Autodesk Inventor part; units mm, degrees
ref_plane "YZ Plane" through (0, 0, 0) normal (1, 0, 0) x (0, 1, 0)
ref_plane "XZ Plane" through (0, 0, 0) normal (0, 1, 0) x (-1, 0, 0)
ref_plane "XY Plane" through (0, 0, 0) normal (0, 0, 1) x (1, 0, 0)
sketch "スケッチ1" plane through (0, 0, 0) normal (0, 1, 0) x (-1, 0, 0)
  line L0 (0, 0) -> (54, 0)
  line L1 (54, 0) -> (54, -66.8)
  line L2 (54, -66.8) -> (0, -66.8)
  line L3 (0, -66.8) -> (0, 0)
  dimension "d0" = 54
  dimension "d1" = 66.8
extrude "押し出し1" add sketch "スケッチ1" along normal blind 10
sketch "スケッチ2" plane through (0, 10, 0) normal (0, 1, 0) x (1, 0, 0)
  line L0 (-54, 66.8) -> (-54, 0)
  line L1 (-54, 0) -> (0, 0)
  line L2 (-27, 0) -> (-27, 66.8)
  line L3 (0, 66.8) -> (-54, 66.8)
  line L4 (-54, 33.4) -> (0, 33.4)
  line L5 (0, 0) -> (0, 66.8)
  line L6 (-27, 33.4) -> (-37.15, 33.4)
  line L7 (-37.15, 33.4) -> (-37.15, 53.55)
  line L8 (-37.15, 53.55) -> (-27, 53.55)
  line L9 (-27, 53.55) -> (-27, 33.4)
  line L10 (-37.15, 33.4) -> (-37.15, 13.25)
  line L11 (-37.15, 13.25) -> (-27, 13.25)
  line L12 (-16.85, 33.4) -> (-16.85, 53.55)
  line L13 (-16.85, 53.55) -> (-27, 53.55)
  line L14 (-16.85, 33.4) -> (-16.85, 13.25)
  line L15 (-16.85, 13.25) -> (-27, 13.25)
  dimension "d7" = 20.15
  dimension "d8" = 10.15
extrude "押し出し2" add sketch "スケッチ2" along normal blind 40 contours L3 L2 L8 L7 L4 L0 | L4 L10 L11 L2 L1 L0 | L3 L5 L4 L12 L13 L2 | L2 L15 L14 L4 L5 L1
fillet "フィレット1" radius 5 4 edges at (0, 25, 0) (0, 25, -66.8) (-54, 25, -66.8) (-54, 25, 0)
sketch "スケッチ3" plane through (0, 0, -5) normal (1, 0, 0) x (0, 0, -1)
  line L0 (48.55, 50) -> (8.25, 50)
  line L1 (28.4, 50) -> (28.4, 0)
  line L2 (0, 0) -> (56.8, 0)
  line L3 (18.4, 50) -> (18.4, 0)
  line L4 (0, 50) -> (0, 0)
  line L5 (0, 10) -> (62, 10)
  line L6 (8.25, 10) -> (48.55, 10)
  point P0 (-5, 0)
  point P1 (18.4, 20)
  point P2 (18.4, 40)
  point P3 (38.4, 20)
  point P4 (38.4, 40)
  dimension "d12" = 10
  dimension "d13" = 10
  dimension "d14" = 10
  dimension "d15" = 20
hole "穴1" at (0, 20, -23.4) at (0, 40, -23.4) at (0, 40, -43.4) at (0, 20, -43.4) direction (-1, 0, 0) diameter 3.3 end through all
sketch "スケッチ4" plane through (0, 0, 0) normal (0, -1, 0) x (1, 0, 0)
  line L0 (-5, -66.8) -> (-49, -66.8)
  line L1 (-27, -66.8) -> (-27, 0)
  line L2 (-49, 0) -> (-5, 0)
  line L3 (-54, -61.8) -> (-54, -5)
  line L4 (-54, -33.4) -> (0, -33.4)
  line L5 (0, -5) -> (0, -61.8)
  point P0 (0, 0)
  point P1 (-27, -43.4)
  point P2 (-27, -23.4)
  dimension "d23" = 10
  dimension "d24" = 10
hole "穴2" at (-27, 0, -43.4) at (-27, 0, -23.4) direction (0, 1, 0) diameter 4.1 end through all
fillet "フィレット2" radius 1 4 edges at (-37.15, 50, -33.4) (-27, 50, -13.25) (-16.85, 50, -33.4) (-27, 50, -53.55)
sketch "スケッチ5" plane through (0, 0, 0) normal (0, -1, 0) x (1, 0, 0)
  circle A0 centre (-27, -23.4) radius 2.05
  circle A1 centre (-27, -43.4) radius 2.05
  line L0 (-27, -23.4) -> (-27, -43.4)
  line L1 (-27, -33.4) -> (-18, -33.4)
  line L2 (-18, -33.4) -> (-18, -40.4)
  line L3 (-18, -40.4) -> (-27, -40.4)
  line L4 (-27, -40.4) -> (-27, -33.4)
  line L5 (-18, -33.4) -> (-18, -26.4)
  line L6 (-18, -26.4) -> (-27, -26.4)
  line L7 (-36, -33.4) -> (-36, -40.4)
  line L8 (-36, -40.4) -> (-27, -40.4)
  line L9 (-36, -33.4) -> (-36, -26.4)
  line L10 (-36, -26.4) -> (-27, -26.4)
  point P0 (0, 0)
  dimension "d33" = 7
  dimension "d34" = 9
extrude "押し出し3" cut sketch "スケッチ5" against normal blind 10 contours L6 L5 L1 L0 | L0 L8 L7 L9 L10 | L1 L2 L3 L0
properties part number "framefixpart1_v2"
Work out the finished part from the listing and answer in its coordinate system (mm). A direction names the side the tool comes from. Coordinates: 2 decimals unless noted, no trailing zeros. Order: outer loops, then holes, each group sorted by start corner. A loop starts at its lowest first (then second) coordinate and runs counter-clockwise, first axis right, second up. Notation, with made-up numbers: (25, -29.5) - (52, -29.5) arc R13 ccw to (52, -6.5) - close; hole circle Ø7 at (78, 74.5). An arc over 180 degrees is marked (long way). Answer as a JSON object with one key per item and string values.
1. The mould has two halves that part along Z. Classify faces 4 (the face through (-45.69, 38.61, -24.29)), 5 (the face through (-27, 25, 0)), 6 (the face through (-17.8, 10, -33.1)), 7 (the face through (-1.43, 25.35, -65.3)): +Z half, -Z half, draft (parallel to the pull), parting line (faces both ways), or undercut.
Output values:
{"face 4": "undercut", "face 5": "+Z half", "face 6": "undercut", "face 7": "-Z half"}
2. Find section C-C on x = -27. Determine the outline of the cut face in (y, z), plus the area to 3 significant figures.
Output values:
{"outline": "(0, -66.8) - (50, -66.8) - (50, -54.55) arc R1 ccw to (49, -53.55) - (10, -53.55) - (10, -45.45) - (0, -45.45) - close; (0, -41.35) - (10, -41.35) - (10, -40.4) - (0, -40.4) - close; (0, -26.4) - (10, -26.4) - (10, -25.45) - (0, -25.45) - close; (0, -21.35) - (10, -21.35) - (10, -13.25) - (49, -13.25) arc R1 ccw to (50, -12.25) - (50, 0) - (0, 0) - close", "area": "1,510 mm²"}
3. Find section A-A on y = 20. Determine the outline of the cut face in (x, z), plus the area to 3 significant figures.
Output values:
{"outline": "(-54, -61.8) arc R5 ccw to (-49, -66.8) - (-5, -66.8) arc R5 ccw to (0, -61.8) - (0, -45.05) - (-16.85, -45.05) - (-16.85, -53.55) - (-37.15, -53.55) - (-37.15, -45.05) - (-54, -45.05) - close; (-54, -41.75) - (-37.15, -41.75) - (-37.15, -25.05) - (-54, -25.05) - close; (-54, -21.75) - (-37.15, -21.75) - (-37.15, -13.25) - (-16.85, -13.25) - (-16.85, -21.75) - (0, -21.75) - (0, -5) arc R5 ccw to (-5, 0) - (-49, 0) arc R5 ccw to (-54, -5) - close; (-16.85, -41.75) - (0, -41.75) - (0, -25.05) - (-16.85, -25.05) - close", "area": "2,550 mm²"}
4. A tool of negligible diameter and unlimited length cuts with its end or side. For faces 1 (the face through (-27, 29, -53.55)), 2 (the face through (-8.54, 38.61, -24.29)), 3 (the face through (-27, 5, -26.4)), from which of +Z, -Z, +X, -X, +Y, -Y can it reach the whole face along a straight path? Write none if from no direction.
Output values:
{"face 1": "+Y", "face 2": "+X, -X", "face 3": "+Y, -Y"}
5. Find section B-B on z = -27.5. Determine the outline of the cut face in (x, y).
Output values:
{"outline": "(-54, 0) - (-36, 0) - (-36, 10) - (-37.15, 10) - (-37.15, 49) arc R1 ccw to (-38.15, 50) - (-54, 50) - close; (-18, 0) - (0, 0) - (0, 50) - (-15.85, 50) arc R1 ccw to (-16.85, 49) - (-16.85, 10) - (-18, 10) - close"}
6. Find section D-D on z = -43.4. Count the separate pieces of the cut face and the enclosed holes in it, plus the area to 3 significant figures.
Output values:
{"separate pieces": "6", "enclosed holes": "0", "area": "1,620 mm²"}
7. Each of these flat-tipped pins is pushed along its axis until it touches: P1, Ø3, axis at y = 20, z = -23.4, coming from the -X side; P2, Ø10, axis at x = -27, z = -35.5, coming from the +Y side. Where does it stop, or does it pass through?
Output values:
{"P1": "passes through", "P2": "stops at y = 10"}
8. Consider line 1 (Y direction, x = -45.75, z = -23.4); line 2 (Z direction, x = -40.75, y = 40); line 3 (X direction, y = 15.5, z = -46). Determine where each line is inside the solid, lowest interval first.
Output values:
{"line 1": "y = 0 to 18.35, 21.65 to 38.35, 41.65 to 50", "line 2": "z = -66.8 to -45.05, -41.75 to -25.05, -21.75 to 0", "line 3": "x = -54 to -37.15, -16.85 to 0"}
